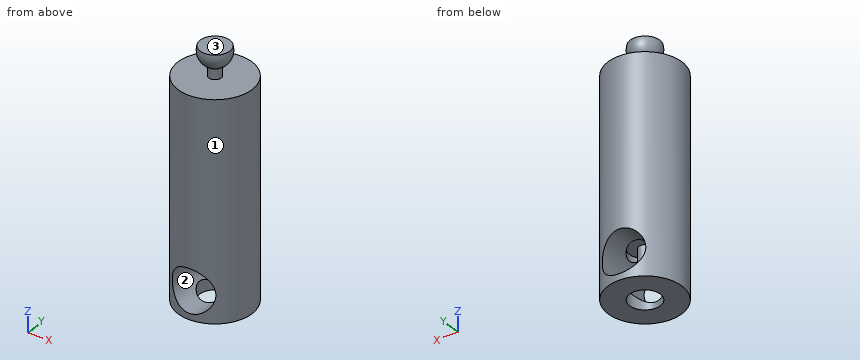
from build123d import *

# Parameters (mm, degrees)
ESQUISSE1_R             = 6
BASE_EXTRUSION_DEPTH    = 35
ESQUISSE2_R             = 3.5
ENL_V_MAT_EXTRU_1_DEPTH = 17.5
ESQUISSE3_R             = 2.5
ENL_V_MAT_EXTRU_2_DEPTH = 8
ESQUISSE4_R             = 1
BOSS_EXTRU_1_DEPTH      = 3.5


with BuildPart() as part:
    # Esquisse1 → Base-Extrusion (new body)
    with BuildSketch(Plane.XY):
        Circle(ESQUISSE1_R)
    extrude(amount=BASE_EXTRUSION_DEPTH)

    # Esquisse2 → Enlèv. mat.-Extru.1 (cut, symmetric)
    with BuildSketch(Plane(origin=(0, 0, 0), x_dir=(1, 0, 0), z_dir=(0, 1, 0))):
        with Locations(Location((0, -4.5, 0), (0, 0, 270))):
            Circle(ESQUISSE2_R)
    extrude(amount=ENL_V_MAT_EXTRU_1_DEPTH, both=True, mode=Mode.SUBTRACT)

    # Esquisse3 → Enlèv. mat.-Extru.2 (cut)
    with BuildSketch(Plane(origin=(0, 0, 0), x_dir=(-1, 0, 0), z_dir=(0, 0, -1))):
        Circle(ESQUISSE3_R)
    extrude(amount=-ENL_V_MAT_EXTRU_2_DEPTH, mode=Mode.SUBTRACT)

    # Esquisse4 → Boss.-Extru.1 (add)
    with BuildSketch(Plane(origin=(0, 0, 8), x_dir=(-1, 0, 0), z_dir=(0, 0, -1))):
        Circle(ESQUISSE4_R)
    extrude(amount=BOSS_EXTRU_1_DEPTH)

    # Esquisse5 → Boss.-Révol.1 (revolve)
    with BuildSketch(Plane(origin=(0, 0, 0), x_dir=(0, 0, -1), z_dir=(1, 0, 0))):
        with BuildLine():
            Line((-35, 1), (-36.708712153, 1))
            ThreePointArc((-36.708712153, 1), (-37.938114865, 2.263271959), (-39.69545069, 2.401322206))
            Line((-39.69545069, 2.401322206), (-39.69545069, 0))
            Line((-39.69545069, 0), (-35, 0))
            Line((-35, 0), (-35, 1))
        make_face()
    revolve(axis=Axis((0, 0, 31.912682492), (0, 0, 1)))


solid = part.part
Input: part model. Units: mm. Frame: model coordinates. Face numbers are marked on the shaded views. Round coordinates to 2 decimals unless told otherwise and drop trailing zeros. Order: outer loops, then holes, each group sorted by start corner. A loop starts at its lowest first (then second) coordinate and runs counter-clockwise, first axis right, second up.
1. Cut plane D-D, the plane z = 34. Output: boundary loops of the cut face in (x, y).
The answers:
outline: circle Ø12 at (0, 0)
2. Mould query, pull axis X, two halves, no side actions, for the marked faces 1, 2 and 3. Classes: released by +X, released by -X, zero draft, split by the parting line, or undercut.
The answers:
face 1: split by the parting line
face 2: undercut
face 3: zero draft
3. Cut plane B-B, the plane y = -1.75. Output: boundary loops of the cut face in (x, z).
The answers:
outline: (-5.74, 0) - (-1.79, 0) - (-1.79, 1.49) arc R3.5 cw to (-1.79, 7.51) - (-1.79, 8) - (1.79, 8) - (1.79, 7.51) arc R3.5 cw to (1.79, 1.49) - (1.79, 0) - (5.74, 0) - (5.74, 35) - (-5.74, 35) - close; (-1.64, 39.7) arc R1.79 ccw (long way) to (1.64, 39.7) - close
4. Cut plane C-C, the plane x = -3. Output: boundary loops of the cut face in (y, z).
The answers:
outline: (-5.2, 0) - (5.2, 0) - (5.2, 2.7) - (-5.2, 2.7) - close; (-5.2, 6.3) - (5.2, 6.3) - (5.2, 35) - (-5.2, 35) - close
5. Cut plane A-A, the plane y = 0. Output: boundary loops of the cut face in (x, z).
The answers:
outline: (-6, 0) - (-2.5, 0) - (-2.5, 2.05) arc R3.5 cw to (-2.5, 6.95) - (-2.5, 8) - (-1, 8) - (-1, 4.5) - (1, 4.5) - (1, 8) - (2.5, 8) - (2.5, 6.95) arc R3.5 cw to (2.5, 2.05) - (2.5, 0) - (6, 0) - (6, 35) - (1, 35) - (1, 36.71) arc R2.5 ccw to (2.4, 39.7) - (-2.4, 39.7) arc R2.5 ccw to (-1, 36.71) - (-1, 35) - (-6, 35) - close
6. Material intervals for line 1 (Z direction, x = 0.25, y = -3); line 2 (Y direction, x = 0, z = 0.9); line 3 (X direction, y = 5.25, z = 7.5), sorted ascending.
The answers:
line 1: z = 0 to 1.01, 7.99 to 35
line 2: y = -6 to -2.5, 2.5 to 6
line 3: x = -2.9 to -1.8, 1.8 to 2.9
7. Pin query (flat end, axial travel): P1, Ø1.5, axis at y = 3.5, z = 32.5, coming from the +X side; P2, Ø1.5, axis at x = -1, y = -1, coming from the -Z side; P3, Ø3, axis at x = -3, z = 28, coming from the +Y side. Return the tip coordinate at first contact, or that it passes through.
The answers:
P1: stops at x = 5.33
P2: stops at z = 4.5
P3: stops at y = 5.81
